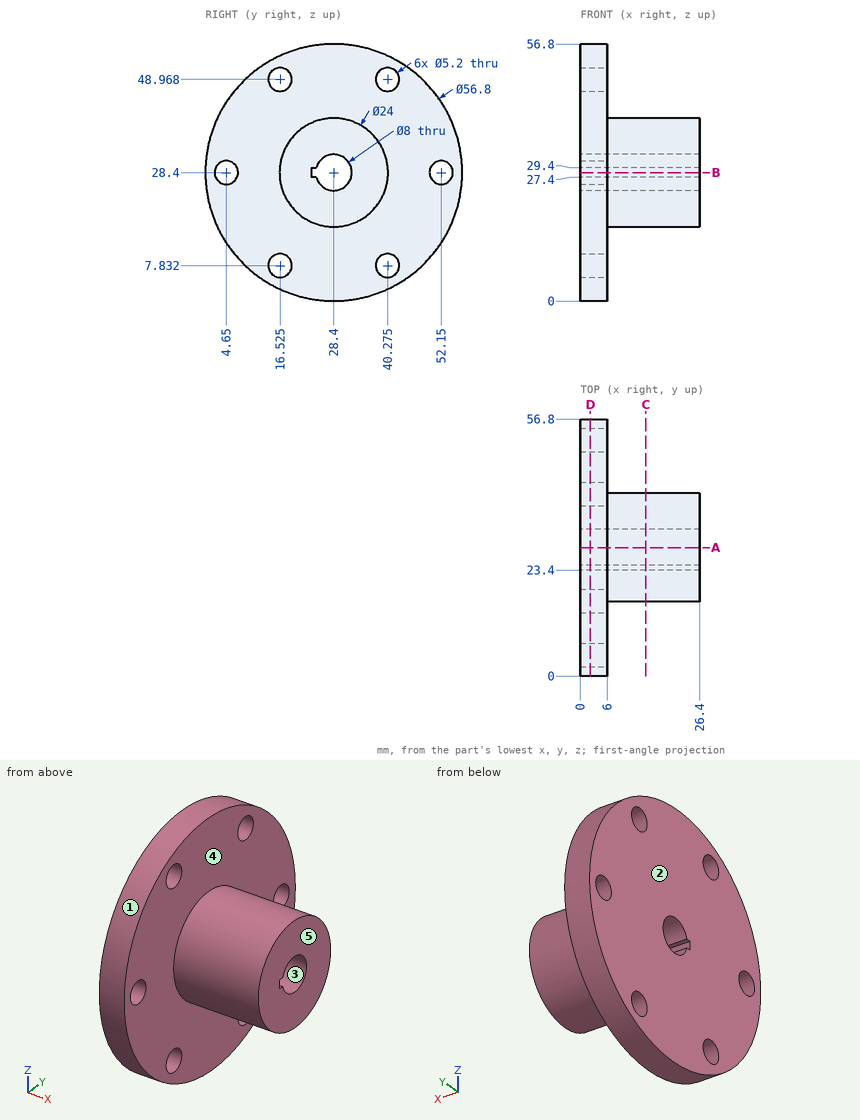
Part print with two shaded views. Sizes in mm from the minimum x, y, z corner. A direction names the side the tool comes from. Give positions to 0.01 mm unless a question says otherwise; leave off trailing zeros. Order: outer loops, then holes, each group sorted by start corner. A loop starts at its lowest first (then second) coordinate and runs counter-clockwise, first axis right, second up. Notation, with made-up numbers: (-27.5, 13.5) - (11.5, 13.5) arc R4 ccw to (11.5, 19.5) - close; hole circle Ø5 at (48.5, -16.75). An arc over 180 degrees is marked (long way). Write each question's results on one line, items separated by ' | '.
1. Saw through at C-C on x = 14.5. List the corners of the cut face in (y, z), and give its area (3 significant figures).
Calculated:
outline: circle Ø24 at (28.4, 28.4); hole (23.4, 27.4) - (24.53, 27.4) arc R4 ccw (long way) to (24.53, 29.4) - (23.4, 29.4) - close | area: 400 mm2
2. Saw through at B-B on z = 28.4. List the corners of the cut face in (x, y), and give its area (3 significant figures).
Calculated:
outline: (0, 0) - (6, 0) - (6, 2.05) - (0, 2.05) - close; (0, 7.25) - (6, 7.25) - (6, 16.4) - (26.4, 16.4) - (26.4, 23.4) - (0, 23.4) - close; (0, 32.4) - (26.4, 32.4) - (26.4, 40.4) - (6, 40.4) - (6, 49.55) - (0, 49.55) - close; (0, 54.75) - (6, 54.75) - (6, 56.8) - (0, 56.8) - close | area: 530 mm2
3. Saw through at A-A on y = 28.4. List the corners of the cut face in (x, z).
Calculated:
outline: (0, 0) - (6, 0) - (6, 16.4) - (26.4, 16.4) - (26.4, 24.4) - (0, 24.4) - close; (0, 32.4) - (26.4, 32.4) - (26.4, 40.4) - (6, 40.4) - (6, 56.8) - (0, 56.8) - close
4. Saw through at D-D on x = 2.25. List the corners of the cut face in (y, z) (3 decimals), and give its area (3 significant figures).
Calculated:
outline: circle Ø56.8 at (28.4, 28.4); hole circle Ø5.2 at (4.65, 28.4); hole circle Ø5.2 at (16.525, 7.832); hole circle Ø5.2 at (16.525, 48.968); hole (23.4, 27.4) - (24.527, 27.4) arc R4 ccw (long way) to (24.527, 29.4) - (23.4, 29.4) - close; hole circle Ø5.2 at (40.275, 7.832); hole circle Ø5.2 at (40.275, 48.968); hole circle Ø5.2 at (52.15, 28.4) | area: 2,350 mm2
5. 3-axis set-ups, long thin cutter, end or side, ignore diameter. For the marked faces 4 and 5: which of +Z, -Z, +X, -X, +Y, -Y reach the whole face in a straight line?
Calculated:
face 4: +X | face 5: +Z, -Z, +X, +Y, -Y
6. Pull direction Z, two halves, no side cores. Call the marked faces 1, 2 and 3: released by +Z, released by -Z, zero draft, split by the parting line, or undercut.
Calculated:
face 1: split by the parting line | face 2: zero draft | face 3: undercut
7. Probe L1, parallel to Y at x = 12.25, z = 28.4; L2, parallel to Y at x = 3.75, z = 50.5; L3, parallel to X at y = 15, z = 26.5. List the from-to ranges inside material, lowest first. Write a range as from..to.
Calculated:
L1: y = 16.4..23.4, 32.4..40.4 | L2: y = 10.56..14.42, 18.63..38.17, 42.38..46.24 | L3: x = 0..6
8. Pin check, flat tips, straight feed: pin 1 (8 mm diameter, centred on x = 20, z = 26.5, fed in from -Y); pin 2 (4 mm diameter, centred on y = 40.28, z = 48.97, fed in from +X); pin 3 (5 mm diameter, centred on x = 12, z = 34, fed in from +Y); pin 4 (7 mm diameter, centred on y = 4.65, z = 28.4, fed in from +X). Stop position of each tip, or through.
Calculated:
pin 1: stops at y = 16.4 | pin 2: passes through | pin 3: stops at y = 39.99 | pin 4: stops at x = 6
